Autodesk Inventor part; units mm, degrees
ref_plane "Work Plane3" through (46, 0, -13.75) normal (-0.8365, 0.5, -0.2241) x (0.2588, 0, -0.9659)
ref_plane "YZ Plane" through (0, 0, 0) normal (1, 0, 0) x (0, 1, 0)
ref_plane "XZ Plane" through (0, 0, 0) normal (0, 1, 0) x (-1, 0, 0)
sketch "Sketch1" plane through (0, 0, 0) normal (0, 0, 1) x (1, 0, 0)
  circle A0 centre (0, 0) radius 5
  circle A1 centre (0, 0) radius 8.45
  arc A2 (-35.8357, 28.841) -> (-35.8357, -28.841) centre (0, 0) ccw
  arc A3 (-28.841, -35.8357) -> (28.841, -35.8357) centre (0, 0) ccw
  circle A4 centre (0, 0) radius 42.5
  circle A5 centre (0, 0) radius 45 construction
  arc A6 (28.0933, -35.1535) -> (35.1535, -28.0933) centre (31.8198, -31.8198) ccw
  circle A7 centre (31.8198, -31.8198) radius 1.45
  arc A8 (35.8357, -28.841) -> (35.8357, 28.841) centre (0, 0) ccw
  circle A9 centre (-31.8198, -31.8198) radius 1.45
  arc A10 (-35.1535, -28.0933) -> (-28.0933, -35.1535) centre (-31.8198, -31.8198) ccw
  circle A11 centre (-31.8198, 31.8198) radius 1.45
  arc A12 (-28.0933, 35.1535) -> (-35.1535, 28.0933) centre (-31.8198, 31.8198) ccw
  line L0 (-31.8198, 31.8198) -> (31.8198, 31.8198) construction
  arc A13 (28.841, 35.8357) -> (-28.841, 35.8357) centre (0, 0) ccw
  circle A14 centre (31.8198, 31.8198) radius 1.45
  arc A15 (35.1535, 28.0933) -> (28.0933, 35.1535) centre (31.8198, 31.8198) ccw
  point P0 (0, -46)
  point P1 (0, 46)
  dimension "d2" = 10
  dimension "d3" = 16.9
  dimension "d4" = 85
  dimension "d5" = 90
  dimension "d6" = 2.9
  dimension "d7" = 5
  dimension "d8" = 360
  dimension "d9" = 92
extrude "Extrusion1" add sketch "Sketch1" against normal blind 2.5 contours A1
extrude "Extrusion2" add sketch "Sketch1" against normal blind 7.5 contours A4
extrude "Extrusion3" add sketch "Sketch1" against normal blind 13.75 contours A12 A13 A15 A8 A6 A3 A10 A2
sketch "Sketch2" plane through (0, 0, -13.75) normal (0, 0, -1) x (-1, 0, 0)
  arc A0 (-35.8357, 28.841) -> (-35.8357, -28.841) centre (0, 0) ccw
  line L0 (-46, 0) -> (-46, -31.8198) construction
  point P0 (-31.8198, -31.8198)
ref_plane "Work Plane1" through (46, 0, -13.75) normal (-0.9659, 0, -0.2588) x (0, -1, 0)
sketch "Sketch3" plane through (46, 0, -13.75) normal (-0.9659, 0, -0.2588) x (0, -1, 0)
  line L0 (0, 0) -> (0, -10) construction
  point P0 (0, 11.9057)
  dimension "d21" = 10
ref_plane "Work Plane3" through (46, 0, -13.75) normal (-0.8365, 0.5, -0.2241) x (0.2588, 0, -0.9659)
sketch "Sketch5" plane through (46, 0, -13.75) normal (-0.8365, 0.5, -0.2241) x (0.2588, 0, -0.9659)
  circle A0 centre (0, 0) radius 5.325
  point P0 (-25.1872, 20.4369)
  dimension "d23" = 10.65
extrude "Extrusion5" cut sketch "Sketch5" along normal mid plane 20
properties part number "Case Part 2 - V2"
Source: CAD feature listing. Evaluate the final solid. Frame: model axes, mm. A direction names the side the tool comes from. Coordinates: 2 decimals unless noted, no trailing zeros. Order: outer loops, then holes, each group sorted by start corner. A loop starts at its lowest first (then second) coordinate and runs counter-clockwise, first axis right, second up. Notation, with made-up numbers: M -22,7 L -18,7 A34 cw -18,43 Z; hole C -8.5,70.5 d4. An arc over 180 degrees is marked long. Write each question's results on one line, items separated by ' | '. Start each with the question number.
Item 1: Set-up query: faces 1 (the face through (-33.727, -25.861, -10.581)), 2 (the face through (46, 0, -7)). Return all of +Z, -Z, +X, -X, +Y, -Y with unobstructed straight access to the full face (end or side cutting, diameter ignored); none if empty.
Item 2: Cut plane C-C (x = -16). Return loops of the section in (y, z).
Item 3: Draft query along Y for faces 3 (the face through (4, -4, -2.5)), 4 (the face through (31.631, 33.257, -6.779)), 5 (the face through (-20.8, -37.3, -13.75)), 6 (the face through (0, 46, -7)). Return one class per face: pulls with the +Y half, pulls with the -Y half, needs draft (parallel to the pull), parting line crosses it, or undercut.
Item 4: Line query: probe 1 along X at (y, z) = (-21.5, -11.5); probe 2 along Y at (x, z) = (10, -9); probe 3 along Z at (x, y) = (-28, 20). Output: solid intervals per line, ascending.
Item 5: First-contact query: pin 1 Ø2 at (y, z) = (6, -5.5) entering from +X; pin 2 Ø8 at (x, z) = (11, -8) entering from +Y; pin 3 Ø2 at (y, z) = (-21, -7.5) entering from +X; pin 4 Ø8 at (x, y) = (0, 0) entering from +Z. Flat tips, straight axial feed; report the tip coordinate or a pass-through.
Item 6: Cut plane B-B (y = -24.5). Return loops of the section in (x, z).
Item 7: Cut plane A-A (x = 0). Return loops of the section in (y, z).
Item 8: Cut plane D-D (z = -5.75). Return loops of the section in (x, y), and give its area (3 significant figures).
Checked values:
1) face 1: -Z | face 2: +Z, -Z, +X
2) outline: M -43.13,-13.75 L -39.37,-13.75 L -39.37,-7.5 L 39.37,-7.5 L 39.37,-13.75 L 43.13,-13.75 L 43.13,0 L -43.13,0 Z
3) face 3: undercut | face 4: undercut | face 5: needs draft | face 6: pulls with the +Y half
4) probe 1: x = -40.67 to -36.66, 36.66 to 40.67 | probe 2: y = -44.9 to -41.31, 41.31 to 44.9 | probe 3: z = -7.5 to 0
5) pin 1: stops at x = 45.73 | pin 2: stops at y = 45.46 | pin 3: stops at x = 41.42 | pin 4: passes through
6) outline: M -38.93,-13.75 L -34.73,-13.75 L -34.73,-7.5 L 34.73,-7.5 L 34.73,-13.75 L 38.93,-13.75 L 38.93,0 L -38.93,0 Z
7) outline: M -46,-13.75 L -42.5,-13.75 L -42.5,-7.5 L -8.45,-7.5 L -8.45,-2.5 L -5,-2.5 L -5,0 L -46,0 Z; M 5,-2.5 L 8.45,-2.5 L 8.45,-7.5 L 42.5,-7.5 L 42.5,-13.75 L 46,-13.75 L 46,0 L 5,0 Z
8) outline: M -35.84,-28.84 A5 ccw -28.84,-35.84 A46 ccw 28.84,-35.84 A5 ccw 35.84,-28.84 A46 ccw 35.84,28.84 A5 ccw 28.84,35.84 A46 ccw -28.84,35.84 A5 ccw -35.84,28.84 A46 ccw Z; hole C -31.82,-31.82 d2.9; hole C -31.82,31.82 d2.9; hole C 0,0 d16.9; hole C 31.82,-31.82 d2.9; hole C 31.82,31.82 d2.9 | area: 6,520 mm2
